Geometry: final body of the model. Coordinates: model frame, mm. A direction names the side the tool comes from. Round coordinates to 2 decimals unless told otherwise and drop trailing zeros. Loops run counter-clockwise (first coordinate to the right, second up) from the corner with the lowest first, then second, coordinate; pieces in that order, holes last. Notation, with made-up numbers: (88.5, 48.5) - (142.5, 48.5) arc R27 cw to (142.5, 82.5) - close; hole circle Ø2 at (80, 31.5). An arc over 180 degrees is marked (long way). Write item = value, one per line. Start each with the question number.
Item 1: Access query for faces 1 (the flat face through (-31, -34, 57)), 2 (the flat face through (-19, 37, 29)), 3 (the flat face through (-29, -34.19, 2)), 4 (the flat face through (29, -33.19, 21)), 5 (the flat face through (5.88, -10.77, 4.46)). Directions: +Z, -Z, +X, -X, +Y, -Y. A direction counts if a zero-diameter tool reaches every point of the face in a straight line with its end or side. Return the directions, or none.
Item 2: Line query: line 1 (Z direction, x = -29, y = 32.5); line 2 (Z direction, x = 20, y = 4); line 3 (X direction, y = -34, z = 27.5). Output: solid intervals per line, ascending. Write a range as from..to.
Item 3: Section A-A (z = 30.5). Return loops of the section in (x, y).
Item 4: First-contact query: pin 1 (5 mm diameter, centred on x = 16.5, y = -24, fed in from -Z); pin 2 (3 mm diameter, centred on x = -8.27, y = 0, fed in from -Z); pin 3 (4 mm diameter, centred on y = -29.5, z = 10.5, fed in from -X); pin 4 (12.5 mm diameter, centred on x = 6.5, y = -11.5, fed in from -Z). Flat tips, straight axial feed; report the tip coordinate or a pass-through.
Item 5: Section B-B (y = 3.5). Count the separate pieces of the cut face and the enclosed holes in it, plus the area to 3 significant figures.
Item 6: Section D-D (y = 28.5). Return loops of the section in (x, z), plus the area to 3 significant figures.
Item 7: Draft query along Y for faces 6 (the flat face through (7.41, 12.2, 2.46)), 7 (the flat face through (-26.663, 37, 47)), 8 (the cylindrical face through (-28.7, 7.62, 2.38)), 9 (the flat face through (18, 36.01, 9)). Return one class per face: pulls with the +Y half, pulls with the -Y half, needs draft (parallel to the pull), parting line crosses it, or undercut.
from build123d import *

# Parameters (mm, degrees)
PAD_DEPTH       = 5
FILLET_R        = 1
FILLET001_R     = 1
FILLET002_R     = 1
SKETCH001_R     = 1.75
PAD001_DEPTH    = 2
SKETCH002_W     = 61.2
SKETCH002_H     = 76.2
PAD002_DEPTH    = 2
PAD003_DEPTH    = 55
SKETCH004_W     = 35
SKETCH004_H     = 25
SKETCH004_W_2   = 14.2
SKETCH004_H_2   = 19
SKETCH004_W_3   = 51.2
SKETCH004_H_3   = 20
POCKET_DEPTH    = 2
SKETCH005_W     = 14.2
SKETCH005_H     = 19
SKETCH005_W_2   = 51.2
SKETCH005_H_2   = 20
POCKET001_DEPTH = 2
SKETCH006_W     = 66.2
SKETCH006_H     = 22
SKETCH006_H_2   = 17
POCKET002_DEPTH = 2
SKETCH007_W     = 24.2
SKETCH007_H     = 10
SKETCH007_W_2   = 31.5
SKETCH007_H_2   = 12
SKETCH007_R     = 1.25
PAD004_DEPTH    = 2
SKETCH008_W     = 31.5
SKETCH008_H     = 2
PAD005_DEPTH    = 3
PAD006_DEPTH    = 2
SKETCH010_W     = 5
SKETCH010_H     = 3
PAD007_DEPTH    = 2
SKETCH011_W     = 6
SKETCH011_H     = 6
SKETCH011_R     = 1.25
PAD008_DEPTH    = 6
SKETCH012_W     = 2
SKETCH012_H     = 10
PAD009_DEPTH    = 25
SKETCH013_W     = 31.5
SKETCH013_H     = 76.2
POCKET003_DEPTH = 6
SKETCH014_W     = 4
SKETCH014_H     = 5
POCKET004_DEPTH = 0.5
SKETCH015_W     = 4
SKETCH015_H     = 5
POCKET005_DEPTH = 0.5


with BuildPart() as part:
    # Sketch → Pad (new body)
    with BuildSketch(Plane.XY):
        Polygon((28.537386, 0), (-14.268693, 24.714102), (-14.268693, -24.714102), align=None)
        Polygon((24.537386, 0), (-12.268693, 21.25), (-12.268693, -21.25), align=None, mode=Mode.SUBTRACT)
    extrude(amount=PAD_DEPTH)

    # Fillet
    fillet_edges = [part.edges().sort_by_distance(p)[0] for p in [
        (-14.268693, -24.714102, 2.5),
    ]]
    fillet(fillet_edges, radius=FILLET_R)

    # Fillet001
    fillet001_edges = [part.edges().sort_by_distance(p)[0] for p in [
        (28.537386, 0, 2.5),
    ]]
    fillet(fillet001_edges, radius=FILLET001_R)

    # Fillet002
    fillet002_edges = [part.edges().sort_by_distance(p)[0] for p in [
        (-14.268693, 24.714102, 2.5),
    ]]
    fillet(fillet002_edges, radius=FILLET002_R)

    # Sketch001 (on Face1 of Fillet002) → Pad001 (join)
    with BuildSketch(Plane(origin=(0, 0, 0), x_dir=(1, 0, 0), z_dir=(0, 0, -1))):
        Polygon((24.537386, 0), (-12.268693, 21.25), (-12.268693, -21.25), align=None)
        with Locations((4.134347, 7.160898)):
            Circle(SKETCH001_R, mode=Mode.SUBTRACT)
        with Locations((4.134347, -7.160898)):
            Circle(SKETCH001_R, mode=Mode.SUBTRACT)
        with Locations((-8.268693, 0)):
            Circle(SKETCH001_R, mode=Mode.SUBTRACT)
        Polygon((8.537386, 0), (-4.268693, 7.393594), (-4.268693, -7.393594), align=None, mode=Mode.SUBTRACT)
    extrude(amount=-PAD001_DEPTH)

    # Sketch002 (on Face9 of Pad001) → Pad002 (join)
    with BuildSketch(Plane.XY.offset(5)):
        with Locations((-1.062614, -0.09)):
            Rectangle(SKETCH002_W, SKETCH002_H)
        Polygon((-12.268693, 21.25), (-12.268693, -21.25), (24.537386, 0), align=None, mode=Mode.SUBTRACT)
    extrude(amount=PAD002_DEPTH)

    # Sketch003 (on Face21 of Pad002) → Pad003 (join)
    with BuildSketch(Plane.XY.offset(7)):
        Polygon((-31.662614, 38.01), (29.537386, 38.01), (29.537386, -38.19), (-31.662614, -38.19), (-31.662614, -36.19), (27.537386, -36.19), (27.537386, 36.01), (-31.662614, 36.01), align=None)
    extrude(amount=PAD003_DEPTH)

    # Sketch004 (on Face26 of Pad003) → Pocket (cut)
    with BuildSketch(Plane.XZ.offset(38.19)):
        with Locations((10.037386, 19.5)):
            Rectangle(SKETCH004_W, SKETCH004_H)
        with Locations((-19.562614, 19.5)):
            Rectangle(SKETCH004_W_2, SKETCH004_H_2)
        with Locations((-1.062614, 47)):
            Rectangle(SKETCH004_W_3, SKETCH004_H_3)
    extrude(amount=-POCKET_DEPTH, mode=Mode.SUBTRACT)

    # Sketch005 (on Face21 of Pocket) → Pocket001 (cut)
    with BuildSketch(Plane(origin=(0, 38.01, 0), x_dir=(-1, 0, 0), z_dir=(0, 1, 0))):
        Polygon((-24.537386, 32), (-12.537386, 32), (-12.537386, 34), (7.462614, 34), (7.462614, 32), (7.462614, 10), (-24.537386, 10), align=None)
        with Locations((19.562614, 19.5)):
            Rectangle(SKETCH005_W, SKETCH005_H)
        with Locations((1.062614, 47)):
            Rectangle(SKETCH005_W_2, SKETCH005_H_2)
    extrude(amount=-POCKET001_DEPTH, mode=Mode.SUBTRACT)

    # Sketch006 (on Face25 of Pocket001) → Pocket002 (cut)
    with BuildSketch(Plane.YZ.offset(29.537386)):
        with Locations((-0.09, 21)):
            Rectangle(SKETCH006_W, SKETCH006_H)
        with Locations((-0.09, 48.5)):
            Rectangle(SKETCH006_W, SKETCH006_H_2)
    extrude(amount=-POCKET002_DEPTH, mode=Mode.SUBTRACT)

    # Sketch007 (on Face62 of Pocket002) → Pad004 (join)
    with BuildSketch(Plane(origin=(0, 0, 32), x_dir=(1, 0, 0), z_dir=(0, 0, -1))):
        Polygon((-31.662614, 36.19), (27.537386, 36.19), (27.537386, -36.01), (12.537386, -36.01), (12.537386, -26.01), (17.537386, -26.01), (17.537386, 26.19), (-31.662614, 26.19), align=None)
        with Locations((-19.562614, -31.01)):
            Rectangle(SKETCH007_W, SKETCH007_H)
        with Locations((45.287386, -32.01)):
            Rectangle(SKETCH007_W_2, SKETCH007_H_2)
        with Locations((58.037386, -32.91)):
            Circle(SKETCH007_R, mode=Mode.SUBTRACT)
        with Locations((32.037386, -32.91)):
            Circle(SKETCH007_R, mode=Mode.SUBTRACT)
        with Locations((45.287386, 32.19)):
            Rectangle(SKETCH007_W_2, SKETCH007_H_2)
        with Locations((32.037386, 33.09)):
            Circle(SKETCH007_R, mode=Mode.SUBTRACT)
        with Locations((58.037386, 33.09)):
            Circle(SKETCH007_R, mode=Mode.SUBTRACT)
    extrude(amount=-PAD004_DEPTH)

    # Sketch008 (on Face78 of Pad004) → Pad005 (join, symmetric)
    with BuildSketch(Plane.XY.offset(34)):
        with Locations((45.287386, 37.01)):
            Rectangle(SKETCH008_W, SKETCH008_H)
        with Locations((45.287386, -37.19)):
            Rectangle(SKETCH008_W, SKETCH008_H)
    extrude(amount=PAD005_DEPTH, both=True)

    # Sketch009 (on Face31 of Pad005) → Pad006 (join)
    with BuildSketch(Plane.XY.offset(62)):
        Polygon((-31.662614, 36.01), (27.537386, 36.01), (27.537386, -36.19), (-31.662614, -36.19), (-31.662614, -34.19), (-31.662614, -31.19), (-27.662614, -31.19), (-27.662614, -34.19), (25.537386, -34.19), (25.537386, 34.01), (-27.662614, 34.01), (-27.662614, 31.01), (-31.662614, 31.01), (-31.662614, 34.01), align=None)
    extrude(amount=-PAD006_DEPTH)

    # Sketch010 (on Face24 of Pad006) → Pad007 (join)
    with BuildSketch(Plane(origin=(-31.662614, 0, 0), x_dir=(0, -1, 0), z_dir=(-1, 0, 0))):
        with Locations((-33.51, 58.5)):
            Rectangle(SKETCH010_W, SKETCH010_H)
        with Locations((33.69, 58.5)):
            Rectangle(SKETCH010_W, SKETCH010_H)
    extrude(amount=-PAD007_DEPTH)

    # Sketch011 (on Face17 of Pad007) → Pad008 (join)
    with BuildSketch(Plane(origin=(-31.662614, 0, 0), x_dir=(0, -1, 0), z_dir=(-1, 0, 0))):
        with Locations((31.19, 2)):
            Rectangle(SKETCH011_W, SKETCH011_H)
        with Locations((31.19, 2)):
            Circle(SKETCH011_R, mode=Mode.SUBTRACT)
        with Locations((-8.81, 2)):
            Rectangle(SKETCH011_W, SKETCH011_H)
        with Locations((-8.81, 2)):
            Circle(SKETCH011_R, mode=Mode.SUBTRACT)
    extrude(amount=-PAD008_DEPTH)

    # Sketch012 (on Face119 of Pad008) → Pad009 (join)
    with BuildSketch(Plane(origin=(0, 0, 32), x_dir=(1, 0, 0), z_dir=(0, 0, -1))):
        with Locations((-8.462614, 31.19)):
            Rectangle(SKETCH012_W, SKETCH012_H)
        with Locations((-8.462614, -31.01)):
            Rectangle(SKETCH012_W, SKETCH012_H)
    extrude(amount=PAD009_DEPTH)

    # Sketch013 (on Face117 of Pad009) → Pocket003 (cut)
    with BuildSketch(Plane.XY.offset(37)):
        with Locations((45.287386, -0.09)):
            Rectangle(SKETCH013_W, SKETCH013_H)
    extrude(amount=-POCKET003_DEPTH, mode=Mode.SUBTRACT)

    # Sketch014 (on Face126 of Pocket003) → Pocket004 (cut)
    with BuildSketch(Plane.XZ.offset(-31.01)):
        with Locations((-29.662614, 59.5)):
            Rectangle(SKETCH014_W, SKETCH014_H)
    extrude(amount=-POCKET004_DEPTH, mode=Mode.SUBTRACT)

    # Sketch015 (on Face126 of Pocket004) → Pocket005 (cut)
    with BuildSketch(Plane(origin=(0, -31.19, 0), x_dir=(-1, 0, 0), z_dir=(0, 1, 0))):
        with Locations((29.662614, 59.5)):
            Rectangle(SKETCH015_W, SKETCH015_H)
    extrude(amount=-POCKET005_DEPTH, mode=Mode.SUBTRACT)


solid = part.part
Taken from the geometry:
q1.face_1 = -X
q1.face_2 = +Y, -Y
q1.face_3 = -Z, +X, -X, -Y
q1.face_4 = +X
q1.face_5 = none
q2.line_1 = 5..7, 32..34, 60..62
q2.line_2 = 0..7, 32..34
q2.line_3 = -9.46..-7.46, 27.54..29.54
q3.outline = (-31.66, -38.19) - (-7.46, -38.19) - (-7.46, -26.19) - (-9.46, -26.19) - (-9.46, -36.19) - (-31.66, -36.19) - close; (-31.66, 36.01) - (-9.46, 36.01) - (-9.46, 26.01) - (-7.46, 26.01) - (-7.46, 38.01) - (-31.66, 38.01) - close; (24.54, 36.01) - (27.54, 36.01) - (27.54, 33.01) - (29.54, 33.01) - (29.54, 38.01) - (24.54, 38.01) - close; (27.54, -38.19) - (29.54, -38.19) - (29.54, -33.19) - (27.54, -33.19) - close
q4.pin_1 = 5
q4.pin_2 = through
q4.pin_3 = -9.46
q4.pin_4 = 0
q5.separate_pieces = 4
q5.enclosed_holes = 0
q5.area = 195 mm^2
q6.outline = (-31.66, 5) - (29.54, 5) - (29.54, 10) - (27.54, 10) - (27.54, 7) - (-7.46, 7) - (-7.46, 34) - (-31.66, 34) - (-31.66, 32) - (-9.46, 32) - (-9.46, 7) - (-31.66, 7) - close; (12.54, 32) - (29.54, 32) - (29.54, 40) - (27.54, 40) - (27.54, 34) - (12.54, 34) - close; (25.54, 60) - (27.54, 60) - (27.54, 57) - (29.54, 57) - (29.54, 62) - (25.54, 62) - close
q6.area = 287 mm^2
q7.face_6 = pulls with the +Y half
q7.face_7 = needs draft
q7.face_8 = undercut
q7.face_9 = pulls with the -Y half
